Job drawing, mm, ordinate dimensions from the low corner. One solid piece. A direction names the side the tool comes from. Round coordinates to 2 decimals unless told otherwise and drop trailing zeros. Loops run counter-clockwise (first coordinate to the right, second up) from the corner with the lowest first, then second, coordinate; pieces in that order, holes last.
1) Mould opens along Y. For the marked faces 4 and 5 say: +Y half, -Y half, draft (parallel to the pull), parting line (faces both ways), or undercut.
2) Probe line 1 (Y direction, x = 87.5, z = 10.5); line 2 (Y direction, x = 26, z = 15); line 3 (Z direction, x = 46, y = 51). List the from-to ranges inside material, lowest first.
3) Band-saw the part on A-A, the plane y = 32.5. Write the cut outline in (x, z).
4) Band-saw the part on D-D, the plane x = 29.5. Write the cut outline in (y, z), then the cut area to 3 significant figures.
5) Band-saw the part on B-B, the plane x = 52. Write the cut outline in (y, z), then the cut area to 3 significant figures.
6) Band-saw the part on C-C, the plane z = 3. Write the cut outline in (x, y).
7) 3-axis set-ups, long thin cutter, end or side, ignore diameter. For the marked faces 1, 2 and 3: which of +Z, -Z, +X, -X, +Y, -Y reach the whole face in a straight line?
8) Drop flat-ended pins along their axis: P1, Ø8, axis at x = 91, z = 11, coming from the +Y side; P2, Ø5.5, axis at y = 57, z = 3, coming from the -X side; P3, Ø3, axis at x = 30.5, y = 30.5, coming from the -Z side; P4, Ø3, axis at y = 39, z = 12.5, coming from the -X side. Give the stop position or say it passes through.
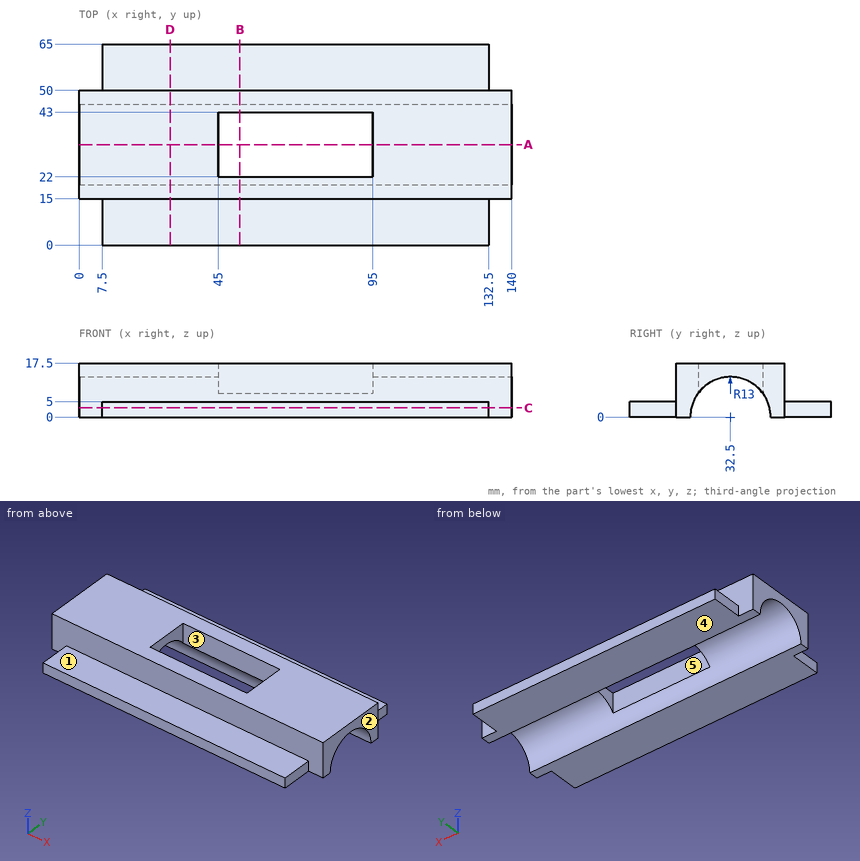
Reported:
1. face 4: draft
1. face 5: undercut
2. line 1: y = 15 to 22, 43 to 50
2. line 2: y = 15 to 50
2. line 3: z = 0 to 5
3. outline: (0, 13) - (45, 13) - (45, 17.5) - (0, 17.5) - close; (95, 13) - (140, 13) - (140, 17.5) - (95, 17.5) - close
4. outline: (0, 0) - (19.5, 0) arc R13 cw to (45.5, 0) - (65, 0) - (65, 5) - (50, 5) - (50, 17.5) - (15, 17.5) - (15, 5) - (0, 5) - close
4. area: 497 mm2
5. outline: (0, 0) - (19.5, 0) arc R13 cw to (22, 7.66) - (22, 17.5) - (15, 17.5) - (15, 5) - (0, 5) - close; (43, 7.66) arc R13 cw to (45.5, 0) - (65, 0) - (65, 5) - (50, 5) - (50, 17.5) - (43, 17.5) - close
5. area: 369 mm2
6. outline: (0, 15) - (7.5, 15) - (7.5, 0) - (132.5, 0) - (132.5, 15) - (140, 15) - (140, 19.85) - (0, 19.85) - close; (0, 45.15) - (140, 45.15) - (140, 50) - (132.5, 50) - (132.5, 65) - (7.5, 65) - (7.5, 50) - (0, 50) - close
7. face 1: +Z, +X, -X, -Y
7. face 2: +Z, -Z, +X, +Y, -Y
7. face 3: +Z, -Z
8. P1: stops at y = 50
8. P2: stops at x = 7.5
8. P3: stops at z = 12.52
8. P4: stops at x = 0
